from build123d import *

# Parameters (mm, degrees)
F1_DEPTH = 10
F3_D     = 5
F4_R     = 1.6
F5_DEPTH = 14.501
F7_R     = 5.5
F8_DEPTH = 10
F9_R     = 4


# Not quite as in the source:
# - an extrude ends at something that could not be found from the text; its depth is read off the source's solid


with BuildPart() as f1:
    # F0 (on Top) → F1 (new body, symmetric)
    with BuildSketch(Plane.XY):
        with BuildLine():
            Line((10, 13), (-10, 13))
            Line((-10, 13), (-10, 0))
            ThreePointArc((-10, 0), (-7.9686887253, -3.9047945105), (-4.5, -6.6143782777))
            Line((-4.5, -6.6143782777), (-4.5, -13))
            Line((-4.5, -13), (-1.5, -13))
            Line((-1.5, -13), (-1.5, -4.9789557138))
            ThreePointArc((-1.5, -4.9789557138), (-3.1016124839, 4.1737273509), (5.2, 0))
            ThreePointArc((5.2, 0), (4.1737273509, -3.1016124839), (1.5, -4.9789557138))
            Line((1.5, -4.9789557138), (1.5, -13))
            Line((1.5, -13), (4.5, -13))
            Line((4.5, -13), (4.5, -6.6143782777))
            ThreePointArc((4.5, -6.6143782777), (7.9686887253, -3.9047945105), (10, 0))
            Line((10, 0), (10, 13))
        make_face()
    extrude(amount=F1_DEPTH, both=True)

    # F3 (through all)
    with Locations(Plane(origin=(0, 13, 0), x_dir=(-1, 0, 0), z_dir=(0, 1, 0))):
        with Locations((0, 0)):
            Hole(F3_D / 2)

    # F4 (on face) → F5 (cut, through all)
    with BuildSketch(Plane(origin=(-4.5, 0, 0), x_dir=(0, -1, 0), z_dir=(-1, 0, 0))):
        with Locations((10, 6)):
            Circle(F4_R)
        with Locations((10, -6)):
            Circle(F4_R)
    extrude(amount=-F5_DEPTH, mode=Mode.SUBTRACT)

    # F7 (on offset) → F8 (cut, through all)
    with BuildSketch(Plane.XZ.offset(-10)):
        Circle(F7_R)
    extrude(amount=F8_DEPTH, mode=Mode.SUBTRACT)

    # F9
    f9_edges = [f1.edges().sort_by_distance(p)[0] for p in [
        (3, -13, 10),
        (-3, -13, 10),
        (-3, -13, -10),
        (3, -13, -10),
    ]]
    fillet(f9_edges, radius=F9_R)


solid = f1.part
Design review of the part built by this model. Coordinates are the model's own, in mm. A direction names the side the tool comes from. Coordinates: 2 decimals unless noted, no trailing zeros. Loops run counter-clockwise (first coordinate to the right, second up) from the corner with the lowest first, then second, coordinate; pieces in that order, holes last.
Item 1: Add section A-A (z = 0). Write out the cut boundary in (x, y), and give its area (3 significant figures).
Completed:
outline: (-10, 0) arc R10.36 ccw to (-4.5, -6.61) - (-4.5, -13) - (-2.5, -13) - (-2.5, -4.56) arc R5.2 cw to (-5.2, 0) - (-5.5, 0) - (-5.5, 10) - (-2.5, 10) - (-2.5, 13) - (-10, 13) - close; (2.5, -13) - (4.5, -13) - (4.5, -6.61) arc R10.36 ccw to (10, 0) - (10, 13) - (2.5, 13) - (2.5, 10) - (5.5, 10) - (5.5, 0) - (5.2, 0) arc R5.2 cw to (2.5, -4.56) - close
area: 217 mm2
Item 2: Draft analysis for pull direction X (two halves, no side actions). For faces 1 (the cylindrical face through (3.021, -11.797, -8.859)), 2 (the flat face through (-3, 10, 0)), 3 (the flat face through (-10, 7, 0)), state which applies: pulls with the +X half, pulls with the -X half, needs draft (parallel to the pull), parting line crosses it, or undercut.
Completed:
face 1: needs draft
face 2: undercut
face 3: pulls with the -X half
Item 3: Add section B-B (x = 0). Write out the cut boundary in (y, z).
Completed:
outline: (5.2, -10) - (13, -10) - (13, -2.5) - (10, -2.5) - (10, -5.5) - (5.2, -5.5) - close; (5.2, 5.5) - (10, 5.5) - (10, 2.5) - (13, 2.5) - (13, 10) - (5.2, 10) - close
Item 4: Add section D-D (x = 3). Write out the cut boundary in (y, z).
Completed:
outline: (-13, -6) arc R4 ccw to (-9, -10) - (-4.25, -10) - (-4.25, 10) - (-9, 10) arc R4 ccw to (-13, 6) - close; (4.25, -10) - (13, -10) - (13, 10) - (4.25, 10) - (4.25, 4.61) - (10, 4.61) - (10, -4.61) - (4.25, -4.61) - close; hole circle Ø3.2 at (-10, -6); hole circle Ø3.2 at (-10, 6)
Item 5: Clearance check with flat-ended pins moving along their axes: pin 1 (4 mm diameter, centred on y = -7.5, z = -7.5, fed in from +X); pin 2 (7 mm diameter, centred on y = -8.5, z = -1, fed in from -X); pin 3 (3.5 mm diameter, centred on y = -10, z = -6, fed in from +X); pin 4 (5.5 mm diameter, centred on x = 1, z = 1, fed in from -Y). State where each tip first meets the part, or that it passes through.
Completed:
pin 1: stops at x = 6.31
pin 2: stops at x = -6.91
pin 3: stops at x = 4.5
pin 4: stops at y = -13
Item 6: Add section C-C (y = -10). Write out the cut boundary in (x, z).
Completed:
outline: (-4.5, -9.87) - (-1.5, -9.87) - (-1.5, -7.6) - (-4.5, -7.6) - close; (-4.5, -4.4) - (-1.5, -4.4) - (-1.5, -2) arc R2.5 cw to (-1.5, 2) - (-1.5, 4.4) - (-4.5, 4.4) - close; (-4.5, 7.6) - (-1.5, 7.6) - (-1.5, 9.87) - (-4.5, 9.87) - close; (1.5, -9.87) - (4.5, -9.87) - (4.5, -7.6) - (1.5, -7.6) - close; (1.5, -4.4) - (4.5, -4.4) - (4.5, 4.4) - (1.5, 4.4) - (1.5, 2) arc R2.5 cw to (1.5, -2) - close; (1.5, 7.6) - (4.5, 7.6) - (4.5, 9.87) - (1.5, 9.87) - close
Item 7: Wall thickness on L1, parallel to X at y = -7, z = 4.75; L2, parallel to X at y = -9.25, z = -1.5; L3, parallel to Z at x = 2.25, y = -10: over which ranges is each line inside the solid? List them lowest first.
Completed:
L1: x = -4.5 to -1.5, 1.5 to 4.5
L2: x = -4.5 to -2, 2 to 4.5
L3: z = -9.87 to -7.6, -4.4 to -1.09, 1.09 to 4.4, 7.6 to 9.87
Item 8: For faces 4 (the cylindrical face through (-8.008, -3.857, 0.14)), 5 (the flat face through (1.5, -8, 6)), 6 (the cylindrical face through (-2.5, -8.8, 0)), 7 (the cylindrical face through (2.5, 6.2, -4.9)), 8 (the flat face through (4.5, -10, 0)), list the 3-axis set-ups (+Z, -Z, +X, -X, +Y, -Y) from which the entire face can be reached by the end or side of a thin tool; tool diameter is ignored.
Completed:
face 4: +Z, -Z, -X, -Y
face 5: +Z, -Z, -Y
face 6: +Y, -Y
face 7: none
face 8: +Z, -Z, +X, -Y
